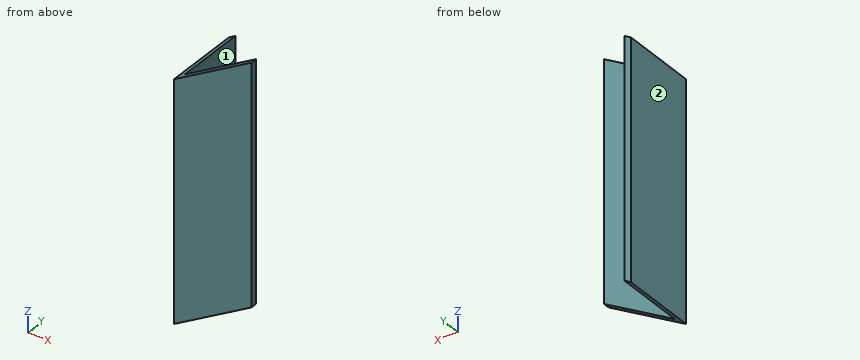
from build123d import *

# Parameters (mm, degrees)
SKETCH1_W           = 38.1
SKETCH1_H           = 38.1
BOSS_EXTRUDE1_DEPTH = 138.43
SKETCH2_W           = 34.925
SKETCH2_H           = 34.925
CUT_EXTRUDE1_DEPTH  = 139.43
CUT_EXTRUDE2_DEPTH  = 38.1


with BuildPart() as part:
    # Sketch1 → Boss-Extrude1 (new body)
    with BuildSketch(Plane.XY):
        with Locations((19.05, 19.05)):
            Rectangle(SKETCH1_W, SKETCH1_H)
    extrude(amount=BOSS_EXTRUDE1_DEPTH)

    # Sketch2 → Cut-Extrude1 (cut, through all)
    with BuildSketch(Plane.XY.offset(138.43)):
        with Locations((20.6375, 20.6375)):
            Rectangle(SKETCH2_W, SKETCH2_H)
    extrude(amount=-CUT_EXTRUDE1_DEPTH, mode=Mode.SUBTRACT)

    # Sketch3 → Cut-Extrude2 (cut)
    with BuildSketch(Plane(origin=(0, 0, 0), x_dir=(-1, 0, 0), z_dir=(0, -1, 0))):
        Polygon((0, 0), (-38.1, 0), (-38.1, -21.997045256), align=None)
        Polygon((0, -138.43), (-38.1, -138.43), (0, -116.432954744), align=None)
    extrude(amount=-CUT_EXTRUDE2_DEPTH, mode=Mode.SUBTRACT)


solid = part.part
Can you work these out from the model? Positions are in its coordinate system, mm. Face numbers are marked on the shaded views. A direction names the side the tool comes from. Give positions to 0.01 mm unless a question says otherwise; leave off trailing zeros. Write each loop counter-clockwise with the first axis right and the second up, starting at its lowest first coordinate (ties: lowest second). Pieces come first, ordered by that corner, then holes. Notation, with made-up numbers: (16, -40) -> (46, -40) arc R31 ccw to (46, -8) -> close; hole circle Ø4 at (24, -3.5). An arc over 180 degrees is marked (long way). Answer as a JSON object with one key per item and string values. Group by question number.
Item 1: Suppose I cut it at A-A (z = 76). Please give me the cut outline in (x, y) (3 decimals).
Item 2: For the marked faces 1 and 2, which set-ups out of +Z, -Z, +X, -X, +Y, -Y let a thin tool reach every point of the face, with its end or its side?
Item 3: I'm going to push flat-ended pins straight in: P1, Ø17.5, axis at x = 16, z = 102.5, coming from the +Y side (3 decimals); P2, Ø2, axis at y = 16.5, z = 66, coming from the +X side (3 decimals); P3, Ø3, axis at x = 21.5, y = 4.5, coming from the +Z side. Where does each tip first touch, or does it pass through?
Item 4: Suppose I cut it at C-C (x = 6.5). Please give me the cut outline in (y, z) (3 decimals).
Item 5: Suppose I cut it at B-B (y = 26.5). Please give me the cut outline in (x, z) (3 decimals), plus the area to 3 significant figures.
Item 6: Please list where these lines run through material, in increasing order: line 1 (Y direction, x = 8.5, z = 92) (3 decimals); line 2 (Z direction, x = 25.5, y = 3). Write a range as [from, to].
Findings:
{
 "1": {"outline": "(0, 0) -> (38.1, 0) -> (38.1, 3.175) -> (3.175, 3.175) -> (3.175, 38.1) -> (0, 38.1) -> close"},
 "2": {"face 1": "+Z, -Z, +X, +Y", "face 2": "+Z, -Z, -X, +Y, -Y"},
 "3": {"P1": "stops at y = 3.175", "P2": "stops at x = 3.175", "P3": "stops at z = 129.25"},
 "4": {"outline": "(0, 3.753) -> (3.175, 3.753) -> (3.175, 120.186) -> (0, 120.186) -> close"},
 "5": {"outline": "(0, 0) -> (3.175, 1.833) -> (3.175, 118.266) -> (0, 116.433) -> close", "area": "370 mm²"},
 "6": {"line 1": "y = [0, 3.175]", "line 2": "z = [14.72, 131.16]"}
}
